from build123d import *

# Parameters (mm, degrees)
F1_DEPTH = 2.54
F2_SIZE  = 2.53999


# Not quite as in the source:
# - a fillet or chamfer is up to 0.001 mm smaller than in the source, because OpenCascade refuses the exact size


with BuildPart() as f1:
    # F0 (on Top) → F1 (new body)
    with BuildSketch(Plane.XY):
        with BuildLine():
            ThreePointArc((-5.5453096033, 4.7335261172), (-3.0532951973, 6.6207338367), (0, 7.2908660733))
            Line((0, 7.2908660733), (0, 52.4203432724))
            Line((0, 52.4203432724), (-4.8945622179, 24.7540763342))
            ThreePointArc((-4.8945622179, 24.7540763342), (-8.3763552073, 20.1468586178), (-14.1500344693, 20.2650334375))
            Line((-14.1500344693, 20.2650334375), (-39.9762034536, 34.1240465641))
            Line((-39.9762034536, 34.1240465641), (-5.5453096033, 4.7335261172))
        make_face()
        with BuildLine():
            Line((0, 52.4203432724), (0, 7.2908660733))
            ThreePointArc((0, 7.2908660733), (3.1432479122, 6.5785044395), (5.6722672278, 4.5806236032))
            Line((5.6722672278, 4.5806236032), (42.2564104309, 34.1240465641))
            Line((42.2564104309, 34.1240465641), (14.255672391, 19.9525133065))
            ThreePointArc((14.255672391, 19.9525133065), (8.5682529825, 19.9287025413), (5.1430312406, 24.46909487))
            Line((5.1430312406, 24.46909487), (0, 52.4203432724))
        make_face()
        with BuildLine():
            ThreePointArc((5.6722672278, 4.5806236032), (6.8743170129, 2.4290931856), (7.2908660733, 0))
            ThreePointArc((7.2908660733, 0), (6.5785044395, -3.1432479122), (4.5806236032, -5.6722672278))
            Line((4.5806236032, -5.6722672278), (31.0746654868, -38.4803079069))
            Line((31.0746654868, -38.4803079069), (18.4844070176, -13.1473843843))
            ThreePointArc((18.4844070176, -13.1473843843), (18.5684546903, -7.3320030677), (23.3522337103, -4.024257286))
            Line((23.3522337103, -4.024257286), (54.3080642819, 0))
            Line((54.3080642819, 0), (26.9017063995, 3.9009043758))
            ThreePointArc((26.9017063995, 3.9009043758), (21.7859881354, 8.139124947), (23.2488130784, 14.6193433195))
            Line((23.2488130784, 14.6193433195), (42.2564104309, 34.1240465641))
            Line((42.2564104309, 34.1240465641), (5.6722672278, 4.5806236032))
        make_face()
        with BuildLine():
            ThreePointArc((4.5806236032, -5.6722672278), (2.4290931856, -6.8743170129), (0, -7.2908660733))
            Line((0, -7.2908660733), (0, -51.5490919352))
            Line((0, -51.5490919352), (2.255521124, -24.8929502638))
            ThreePointArc((2.255521124, -24.8929502638), (6.3641325232, -19.4785950158), (13.0147117735, -20.8806385306))
            Line((13.0147117735, -20.8806385306), (31.0746654868, -38.4803079069))
            Line((31.0746654868, -38.4803079069), (4.5806236032, -5.6722672278))
        make_face()
        with BuildLine():
            Line((0, -51.5490919352), (0, -7.2908660733))
            ThreePointArc((0, -7.2908660733), (-3.1432479122, -6.5785044395), (-5.6722672278, -4.5806236032))
            Line((-5.6722672278, -4.5806236032), (-39.9762034536, -32.2826717697))
            Line((-39.9762034536, -32.2826717697), (-14.4636689781, -16.8901939339))
            ThreePointArc((-14.4636689781, -16.8901939339), (-8.5166009917, -16.5643608756), (-4.9155814374, -21.3084564677))
            Line((-4.9155814374, -21.3084564677), (0, -51.5490919352))
        make_face()
        with BuildLine():
            ThreePointArc((-5.6722672278, -4.5806236032), (-6.8743170129, -2.4290931856), (-7.2908660733, 0))
            Line((-7.2908660733, 0), (-13.3722843602, 0))
            Line((-13.3722843602, 0), (-56.1868394799, 0))
            Line((-56.1868394799, 0), (-25.1595931562, -2.7541493308))
            ThreePointArc((-25.1595931562, -2.7541493308), (-19.7516975402, -6.9137834915), (-21.2347588093, -13.5732444768))
            Line((-21.2347588093, -13.5732444768), (-39.9762034536, -32.2826717697))
            Line((-39.9762034536, -32.2826717697), (-5.6722672278, -4.5806236032))
        make_face()
        with BuildLine():
            Line((-13.3722843602, 0), (-7.2908660733, 0))
            ThreePointArc((-7.2908660733, 0), (-6.8405715313, 2.5225600534), (-5.5453096033, 4.7335261172))
            Line((-5.5453096033, 4.7335261172), (-39.9762034536, 34.1240465641))
            Line((-39.9762034536, 34.1240465641), (-22.9918849286, 13.0920645237))
            ThreePointArc((-22.9918849286, 13.0920645237), (-22.0777388727, 6.6432422744), (-27.3229831249, 2.7818456164))
            Line((-27.3229831249, 2.7818456164), (-56.1868394799, 0))
            Line((-56.1868394799, 0), (-13.3722843602, 0))
        make_face()
    extrude(amount=F1_DEPTH)

    # F2 (size 2.54 in the source; OpenCascade refuses exactly that, so slightly less here)
    f2_edges = [f1.edges().sort_by_distance(p)[0] for p in [
        (28.256041, 27.03828, 2.54),
        (40.604885, 1.950452, 2.54),
        (24.779536, -25.813846, 2.54),
        (22.044689, -29.680473, 2.54),
        (-2.447281, 38.58721, 2.54),
        (-31.484044, 23.608056, 2.54),
        (-30.605481, -22.927958, 2.54),
        (-2.457791, -36.428774, 2.54),
    ]]
    chamfer(f2_edges, length=F2_SIZE)

    # F3: F1 across plane


with BuildPart() as f1_1:
    add(f1.part)
    add(f1.part.mirror(Plane.XY))


solid = f1_1.part
The model under review builds one solid part; all positions refer to its coordinate system, in mm. A direction names the side the tool comes from. Coordinates: 2 decimals unless noted, no trailing zeros. Put each result on its own line as item: value. Start each with the question number.
Q1. For faces 5 (the flat face through (35, -1.5, 1)), 6 (the flat face through (-28.71, 22.23, 1.29)), 7 (the flat face through (0.361, -35.361, -1.006)), 8 (the flat face through (35, -1.5, -1)), list the 3-axis set-ups (+Z, -Z, +X, -X, +Y, -Y) from which the entire face can be reached by the end or side of a thin tool; tool diameter is ignored.
Q2. Clearance check with flat-ended pins moving along their axes: pin 1 (5 mm diameter, centred on x = 25.5, y = 28, fed in from +Z); pin 2 (1 mm diameter, centred on x = 41.5, z = -1, fed in from +Y); pin 3 (2 mm diameter, centred on x = -35, z = 0.5, fed in from -Y). State where each tip first meets the part, or that it passes through.
Q3. Add section B-B (y = 29.5). Count the separate pieces of the cut face and the enclosed holes in it, and give its area (3 significant figures).
Q4. Wall thickness on line 1 (X direction, y = -20.5, z = 1); line 2 (Y direction, x = 30, z = -0.1); line 3 (Y direction, x = -23, z = -1.95): over which ranges is each line inside the solid? List them lowest first.
Q5. The part is to be moulded in two halves that separate along Y. For faces 1 (the conical face through (6.11, -19.104, -0.441)), 2 (the flat face through (25.92, 24.41, 1.29)), 3 (the conical face through (21.403, 7.898, 0.441)), 4 (the flat face through (-37.35, -0.66, -1.01)), say which applies: +Y half, -Y half, draft (parallel to the pull), parting line (faces both ways), or undercut.
Answers:
1. face 5: +Z, +X
1. face 6: +Z, -X
1. face 7: -Z, -Y
1. face 8: -Z, +X
2. pin 1: stops at z = 0.4
2. pin 2: stops at y = 1.32
2. pin 3: stops at y = -29.8
3. separate pieces: 3
3. enclosed holes: 0
3. area: 41.9 mm^2
4. line 1: x = -26.76 to -22.38, -4.06 to 3.13, 14.06 to 21.02
4. line 2: y = -37.29 to -36.54, -3.06 to 3.36, 21.69 to 27.81
4. line 3: y = -19.76 to -18.09, -1.24 to 2.43, 16.21 to 22.8
5. face 1: -Y half
5. face 2: +Y half
5. face 3: undercut
5. face 4: undercut
